For this review, use the dimensioned drawing (mm, ordinates from the lowest corner) and the shaded views. A direction names the side the tool comes from. Give positions to 0.01 mm unless a question says otherwise; leave off trailing zeros. Order: outer loops, then holes, each group sorted by start corner. A loop starts at its lowest first (then second) coordinate and runs counter-clockwise, first axis right, second up. Notation, with made-up numbers: M 63.5,83 L 91.5,83 A32 ccw 91.5,109 Z; hole C 43.25,55 d5. An arc over 180 degrees is marked long. Use CSV: the item, a comma, the result in double quotes. Start each with the question number.
(1) Tool access review of the marked faces 1 and 2: name each direction out of +Z, -Z, +X, -X, +Y, -Y from which nothing blocks a thin tool from reaching the whole face with its end or side.
(2) Consider section D-D (y = 26.5). Write out the cut boundary in (x, z), and give its area (3 significant figures).
(3) Draft analysis for pull direction Y (two halves, no side actions). For the marked faces 3, 4, 5 and 6, state which applies: pulls with the +Y half, pulls with the -Y half, needs draft (parallel to the pull), parting line crosses it, or undercut.
(4) Wall thickness on L1, parallel to X at y = 29.5, z = 11; L2, parallel to Y at x = 16.5, z = 6; L3, parallel to Z at x = 64, y = 9: over which ranges is each line inside the solid? List them lowest first. Write a range as from..to.
(5) Consider section B-B (z = 3). Write out the cut boundary in (x, y), and give its area (3 significant figures).
(6) Consider section C-C (x = 44). Write out the cut boundary in (y, z), and give its area (3 significant figures).
(7) Consider section A-A (z = 24.5). Write out the cut boundary in (x, y).
(8) Clearance check with flat-ended pins moving along their axes: P1, Ø2, axis at x = 47, y = 50.5, coming from the +Z side; P2, Ø1, axis at x = 17, y = 58.5, coming from the +Z side. State where each tip first meets the part, or that it passes through.
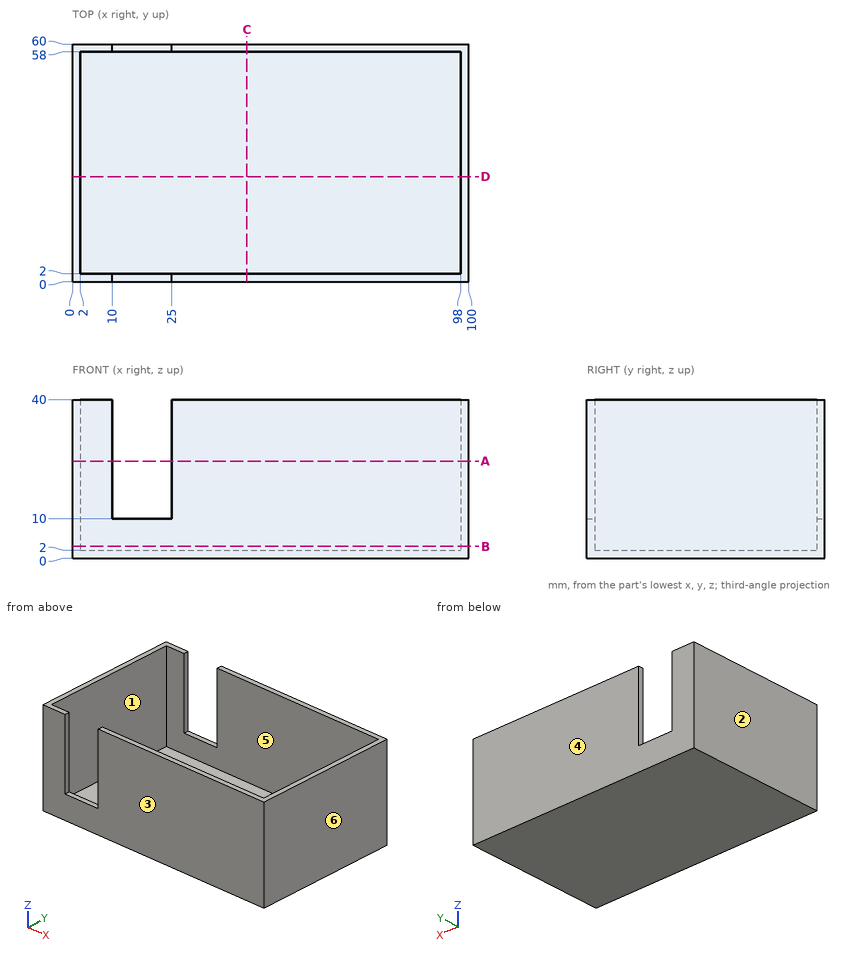
Check result:
1,face 1,"+Z"
1,face 2,"+Z, -Z, -X, +Y, -Y"
2,outline,"M 0,0 L 100,0 L 100,40 L 98,40 L 98,2 L 2,2 L 2,40 L 0,40 Z"
2,area,"352 mm^2"
3,face 3,"pulls with the -Y half"
3,face 4,"pulls with the +Y half"
3,face 5,"undercut"
3,face 6,"needs draft"
4,L1,"x = 0..2, 98..100"
4,L2,"y = 0..2, 58..60"
4,L3,"z = 0..2"
5,outline,"M 0,0 L 100,0 L 100,60 L 0,60 Z; hole M 2,2 L 98,2 L 98,58 L 2,58 Z"
5,area,"624 mm^2"
6,outline,"M 0,0 L 60,0 L 60,40 L 58,40 L 58,2 L 2,2 L 2,40 L 0,40 Z"
6,area,"272 mm^2"
7,outline,"M 0,0 L 10,0 L 10,2 L 2,2 L 2,58 L 10,58 L 10,60 L 0,60 Z; M 25,0 L 100,0 L 100,60 L 25,60 L 25,58 L 98,58 L 98,2 L 25,2 Z"
8,P1,"stops at z = 2"
8,P2,"stops at z = 10"
